from build123d import *

# Parameters (mm, degrees)
F0_W      = 42.4
F0_H      = 40
F0_R      = 1.55
F0_R_2    = 18.5
F0_W_2    = 1.3
F1_DEPTH  = 3.5
F2_W      = 1.3
F2_H      = 40
F3_DEPTH  = 55
F6_D      = 3.5
F6_DEPTH  = 43.701
F7_DEPTH  = 0.7
F8_DEPTH  = 0.7
F9_W      = 20
F9_H      = 7.8327696025
F10_DEPTH = 60
F11_D     = 3.5
F12_R     = 1.6
F13_DEPTH = 60


with BuildPart() as f1:
    # F0 (on Top) → F1 (new body)
    with BuildSketch(Plane.XY):
        with Locations((9.9029783159, 0)):
            Rectangle(F0_W, F0_H)
        with Locations((-6.0970216841, -16)):
            Circle(F0_R, mode=Mode.SUBTRACT)
        with Locations((25.9029783159, -16)):
            Circle(F0_R, mode=Mode.SUBTRACT)
        with Locations((-6.0970216841, 16)):
            Circle(F0_R, mode=Mode.SUBTRACT)
        with Locations((9.9029783159, 0)):
            Circle(F0_R_2, mode=Mode.SUBTRACT)
        with Locations((25.9029783159, 16)):
            Circle(F0_R, mode=Mode.SUBTRACT)
        with Locations((-11.9470216841, 0)):
            Rectangle(F0_W_2, F0_H)
        with Locations((31.7529783159, 0)):
            Rectangle(F0_W_2, F0_H)
    extrude(amount=-F1_DEPTH)

    # F2 (on face) → F3 (join)
    with BuildSketch(Plane.XY):
        with Locations((-11.9470216841, 0)):
            Rectangle(F2_W, F2_H)
        with Locations((31.7529783159, 0)):
            Rectangle(F2_W, F2_H)
    extrude(amount=F3_DEPTH)

    # F6 (through all, one way)
    with BuildSketch(Plane(origin=(-11.2970216841, 0, 0), x_dir=(0, 1, 0), z_dir=(-1, 0, 0))):
        with Locations((5, -50), (-14, -50), (0, -6)):
            Circle(F6_D / 2)
    extrude(amount=-F6_DEPTH, mode=Mode.SUBTRACT)

    # F7 (add): a face of the model
    f7_faces = [f1.faces().sort_by_distance(p)[0] for p in [
        (32.4029783159, 0.0374664773, 25.6303154199),
    ]]
    extrude(f7_faces, amount=F7_DEPTH)

    # F8 (add): a face of the model
    f8_faces = [f1.faces().sort_by_distance(p)[0] for p in [
        (-12.5970216841, 0, 25.75),
    ]]
    extrude(f8_faces, amount=F8_DEPTH)

    # F9 (on face) → F10 (cut)
    with BuildSketch(Plane(origin=(-13.2970216841, 0, 0), x_dir=(0, -1, 0), z_dir=(-1, 0, 0))):
        with Locations((10, 51.0836151987)):
            Rectangle(F9_W, F9_H)
    extrude(amount=-F10_DEPTH, mode=Mode.SUBTRACT)

    # F11 (through all)
    with Locations(Plane(origin=(31.1029783159, 0, 0), x_dir=(0, -1, 0), z_dir=(1, 0, 0))):
        with Locations((-5, -50)):
            Hole(F11_D / 2)

    # F12 (on face) → F13 (cut)
    with BuildSketch(Plane(origin=(-13.2970216841, 0, 0), x_dir=(0, -1, 0), z_dir=(-1, 0, 0))):
        with Locations((0, 6.2575037591)):
            Circle(F12_R)
    extrude(amount=-F13_DEPTH, mode=Mode.SUBTRACT)


solid = f1.part
CAD build for the part. Positions are in the model's coordinates, mm. A direction names the side the tool comes from. Coordinates: 2 decimals unless noted, no trailing zeros. Write each loop counter-clockwise with the first axis right and the second up, starting at its lowest first coordinate (ties: lowest second). Pieces come first, ordered by that corner, then holes. Notation, with made-up numbers: (5.5, 88) - (47.5, 88) arc R32 cw to (47.5, 116) - close; hole circle Ø10 at (-38.5, 81.25). An arc over 180 degrees is marked (long way). Use a Markdown table: item, result. Add a question column.
Item 1: Mould opens along Z. For faces 1 (the face through (-11.297, 0, 27)), 2 (the face through (32.09, 0.06, 4.25)), 3 (the face through (5, -18, -3.5)) say: pulls with the +Z half, pulls with the -Z half, needs draft (parallel to the pull), parting line crosses it, or undercut.
Item 2: Band-saw the part on D-D, the plane y = 4.5. Give the cut face in (x, z).
Item 3: Flat gauge pins, fed straight in: pin 1 (3 mm diameter, centred on y = 0, z = 6, fed in from +X); pin 2 (2.5 mm diameter, centred on x = 25.9, y = -16, fed in from -Z); pin 3 (0.6 mm diameter, centred on x = -12.5, y = -12, fed in from +Z); pin 4 (1 mm diameter, centred on x = -12, z = 49.5, fed in from -Y). Where does each tip first touch, or does it go through?
Item 4: Band-saw the part on C-C, the plane y = -5. Give the cut face in (x, z), and give its area (3 significant figures).
Item 5: Band-saw the part on B-B, the plane x = 21.5. Give the cut face in (y, z), and give its area (3 significant figures).
Item 6: Drill centre lines: L1, parallel to X at y = 18, z = 28.5; L2, parallel to X at y = 16.5, z = -1; L3, parallel to Y at x = -12, z = 50. Where is each one in solid material? Low to high. Write a range as from..to.
Item 7: Band-saw the part on A-A, the plane z = 16.5. Give the cut face in (x, y).
Item 8: 3-axis set-ups, long thin cutter, end or side, ignore diameter. For faces 4 (the face through (32, -10, 47.167)), 5 (the face through (32.089, -0.023, 7.857)), 6 (the face through (10, -20, -1)), 7 (the face through (5, 18, 0)): which of +Z, -Z, +X, -X, +Y, -Y reach the whole face in a straight line?
Numbers:
| question | item | result |
|---|---|---|
| 1 | face 1 | needs draft |
| 1 | face 2 | undercut |
| 1 | face 3 | pulls with the -Z half |
| 2 | outline | (-13.3, -3.5) - (-8.04, -3.5) - (-8.04, 0) - (-11.3, 0) - (-11.3, 48.32) - (-13.3, 48.32) - close; (-13.3, 51.68) - (-11.3, 51.68) - (-11.3, 55) - (-13.3, 55) - close; (27.85, -3.5) - (33.1, -3.5) - (33.1, 48.32) - (31.1, 48.32) - (31.1, 0) - (27.85, 0) - close; (31.1, 51.68) - (33.1, 51.68) - (33.1, 55) - (31.1, 55) - close |
| 3 | pin 1 | x = -11.3 |
| 3 | pin 2 | through |
| 3 | pin 3 | z = 47.17 |
| 3 | pin 4 | y = 0 |
| 4 | outline | (-13.3, -3.5) - (-7.91, -3.5) - (-7.91, 0) - (-11.3, 0) - (-11.3, 47.17) - (-13.3, 47.17) - close; (27.71, -3.5) - (33.1, -3.5) - (33.1, 47.17) - (31.1, 47.17) - (31.1, 0) - (27.71, 0) - close |
| 4 | area | 226 mm2 |
| 5 | outline | (-20, -3.5) - (-14.41, -3.5) - (-14.41, 0) - (-20, 0) - close; (14.41, -3.5) - (20, -3.5) - (20, 0) - (14.41, 0) - close |
| 5 | area | 39.1 mm2 |
| 6 | L1 | -13.3..-11.3, 31.1..33.1 |
| 6 | L2 | -13.3..-7.56, -4.63..1.54, 18.27..24.44, 27.37..33.1 |
| 6 | L3 | 0..3.25, 6.75..20 |
| 7 | outline | (-13.3, -20) - (-11.3, -20) - (-11.3, 20) - (-13.3, 20) - close; (31.1, -20) - (33.1, -20) - (33.1, 20) - (31.1, 20) - close |
| 8 | face 4 | +Z, +X, -X, -Y |
| 8 | face 5 | +X, -X |
| 8 | face 6 | +Z, -Z, +X, -X, -Y |
| 8 | face 7 | +Z, +Y, -Y |
